Geometry: see drawing. Coordinates: mm, zero at the bounding-box minimum. A direction names the side the tool comes from. Give positions to 0.01 mm unless a question says otherwise; leave off trailing zeros. Write each loop counter-clockwise with the first axis right and the second up, starting at its lowest first coordinate (ties: lowest second). Pieces come first, ordered by that corner, then holes. Notation, with made-up numbers: M 14,71.5 L 49,71.5 A22 ccw 49,100.5 Z; hole C 11.5,11 d1. An arc over 180 degrees is marked long. Use a Markdown table: item, result. Add a question column.
1) Section B-B on x = 6.25. Return the cut outline in (y, z).
2) Pin query (flat end, axial travel): pin 1 (1.5 mm diameter, centred on x = 2, y = 12.5, fed in from -Z); pin 2 (7.5 mm diameter, centred on x = 8.5, z = 6, fed in from -Y). Return the tip coordinate at first contact, or that it passes through.
3) Section D-D on z = 4.25. Return the cut outline in (x, y).
4) Section C-C on x = 3.5. Return the cut outline in (y, z).
5) Set-up query: the marked faces 1 and 2. Return all of +Z, -Z, +X, -X, +Y, -Y with unobstructed straight access to the full face (end or side cutting, diameter ignored); none if empty.
6) Section A-A on y = 5. Return the cut outline in (x, z).
7) Line query: line 1 (Z direction, x = 13.5, y = 21); line 2 (Y direction, x = 7.5, z = 16) (1 decimal); line 3 (Y direction, x = 7.5, z = 16.3) (1 decimal). Output: solid intervals per line, ascending.
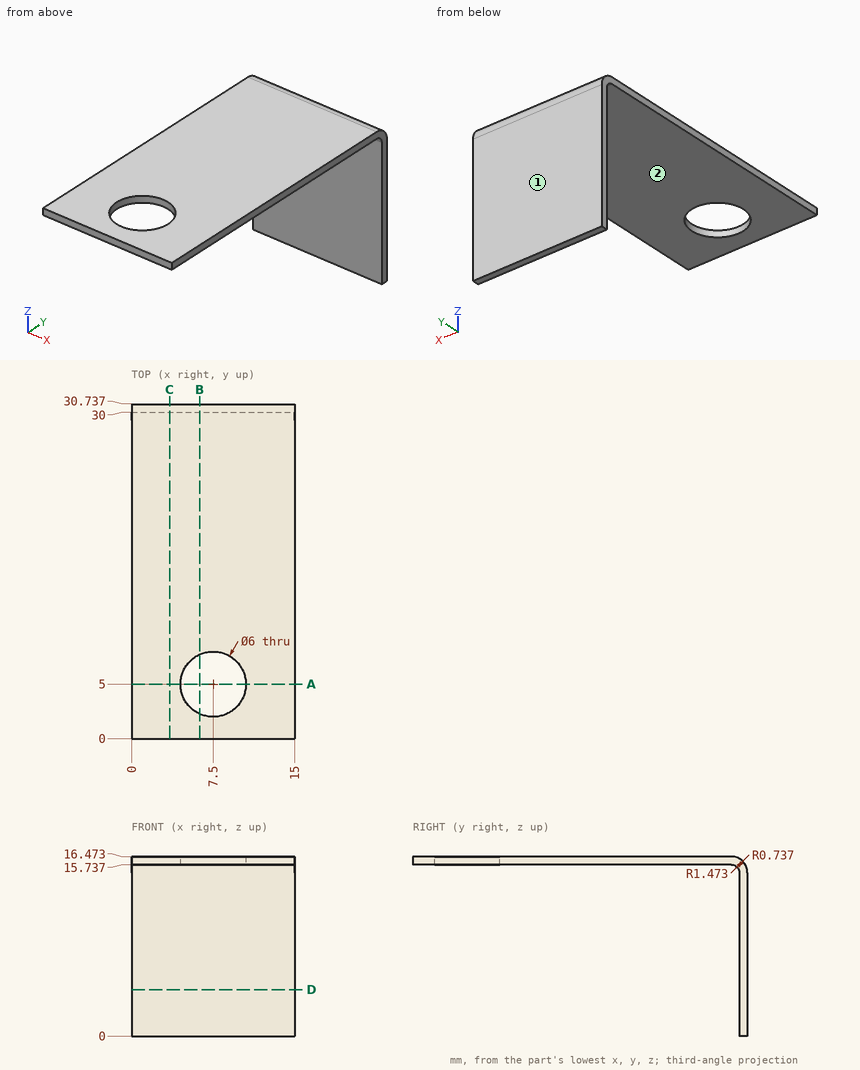
Found:
| question | item | result |
|---|---|---|
| 1 | outline | M 0,15.74 L 2.27,15.74 L 2.27,16.47 L 0,16.47 Z; M 7.73,15.74 L 29.26,15.74 A0.74 cw 30,15 L 30,0 L 30.74,0 L 30.74,15 A1.47 ccw 29.26,16.47 L 7.73,16.47 Z |
| 2 | pin 1 | z = 15.74 |
| 2 | pin 2 | y = 30 |
| 3 | outline | M 0,30 L 15,30 L 15,30.74 L 0,30.74 Z |
| 4 | outline | M 0,15.74 L 29.26,15.74 A0.74 cw 30,15 L 30,0 L 30.74,0 L 30.74,15 A1.47 ccw 29.26,16.47 L 0,16.47 Z |
| 5 | face 1 | +Z, -Z, +X, -X, +Y |
| 5 | face 2 | -Z, +X, -X, -Y |
| 6 | outline | M 0,15.74 L 4.5,15.74 L 4.5,16.47 L 0,16.47 Z; M 10.5,15.74 L 15,15.74 L 15,16.47 L 10.5,16.47 Z |
| 7 | line 1 | 15.74 to 16.47 |
| 7 | line 2 | 0 to 2, 8 to 30.3 |
| 7 | line 3 | 0 to 2, 8 to 30 |
